Autodesk Inventor part; units mm, degrees
ref_plane "開始平面" through (0, 0, 0) normal (0, 0, 1) x (1, 0, 0)
ref_plane "終了平面" through (0, 0, 300) normal (0, 0, 1) x (1, 0, 0)
ref_plane "YZ Plane" through (0, 0, 0) normal (1, 0, 0) x (0, 1, 0)
ref_plane "開始平面" through (0, 0, 0) normal (0, 0, 1) x (1, 0, 0)
ref_plane "終了平面" through (0, 0, 300) normal (0, 0, 1) x (1, 0, 0)
sketch "スケッチ" plane through (0, 0, 0) normal (0, 0, 1) x (1, 0, 0)
  line L0 (-12.8, 0) -> (-12.8, 37.5)
  line L1 (-12.8, 37.5) -> (27.2, 37.5)
  line L2 (27.2, 37.5) -> (27.2, 35.6964)
  line L3 (23.5486, 31.7116) -> (-0.4973, 29.6078)
  line L4 (-7.8, 21.6383) -> (-7.8, 0)
  line L5 (-7.8, 0) -> (-12.8, 0) construction
  line L6 (9.7, 37.5) -> (9.7, 30.5) construction
  line L7 (27.2, 32.0311) -> (27.2, 30.5) construction
  line L8 (27.2, 30.5) -> (9.7, 30.5) construction
  line L9 (0, 15) -> (0, -27) construction
  line L10 (-5.539, 0) -> (16.0067, 0) construction
  line L11 (-12.8, 0) -> (-12.8, -37.5)
  line L12 (-12.8, -37.5) -> (27.2, -37.5)
  line L13 (27.2, -37.5) -> (27.2, -35.6964)
  line L14 (23.5486, -31.7116) -> (-0.4973, -29.6078)
  line L15 (-7.8, -21.6383) -> (-7.8, 0)
  arc A0 (-0.4973, 29.6078) -> (-7.8, 21.6383) centre (0.2, 21.6383) ccw
  arc A1 (-7.8, -21.6383) -> (-0.4973, -29.6078) centre (0.2, -21.6383) ccw
  arc A2 (23.5486, 31.7116) -> (27.2, 35.6964) centre (23.2, 35.6964) ccw
  arc A3 (27.2, -35.6964) -> (23.5486, -31.7116) centre (23.2, -35.6964) ccw
  line L16 (0, 52.5) -> (0, -52.5) construction
  line L17 (-20.955, 0) -> (36.1298, 0) construction
  point P0 (-7.8, 28.9689)
  point P1 (27.2, -32.0311)
  point P2 (-7.8, -28.9689)
  point P3 (9.7, -37.5)
  point P4 (9.7, -30.5)
  dimension "d0" = 5
  dimension "d1" = 37.5
  dimension "d2" = 40
  dimension "d3" = 7
  dimension "d4" = 17.5
  dimension "d5" = 1.5311
  dimension "d23" = 8
  dimension "d24" = 4
  dimension "d25" = 12.8
extrude "ボディ" add sketch "スケッチ" along normal up to surface (300 mm away) from surface at 0
sketch "Sketch3" plane through (0, 0, 0) normal (0, 0, 1) x (1, 0, 0)
  line L0 (0, 0) -> (10, 0)
ref_plane "Work Plane3" through (0, 0, 0) normal (0, -1, 0) x (1, 0, 0)
sketch "Sketch4" plane through (0, 0, 0) normal (0, -1, 0) x (1, 0, 0)
  line L0 (-2, 0) -> (12, 0)
  line L1 (-2, 300) -> (12, 300)
  dimension "d29" = 300
equation "\"d0\" = G_T"
equation "\"d1\" = 0.5 * G_H"
equation "\"d2\" = G_W"
equation "\"d3\" = G_T1"
equation "\"d4\" = G_C"
equation "\"d23\" = G_IR"
equation "\"d24\" = G_ER"
equation "\"d25\" = ey"
equation "\"d6\" = G_L"
equation "\"G_W\" = 40"
equation "\"G_H\" = 75"
equation "\"G_T\" = 5"
equation "\"G_T1\" = 7"
equation "\"G_NG\" = 0.08749"
equation "\"G_ER\" = 4"
equation "\"G_IR\" = 8"
equation "\"G_C\" = 17.5"
equation "\"G_L\" = d29"
equation "\"ey\" = 12.8"
equation "\"G_OFFSET_START\" = 0"
equation "\"G_OFFSET_END\" = 0"
properties part number "JIS G 3192 - 75 x 40 x 5 - 300" material "SS400"
Geometry check sheet. Reference: the model listing, model coordinates, mm. A direction names the side the tool comes from. Give positions to 0.01 mm unless a question says otherwise; leave off trailing zeros. Order: outer loops, then holes, each group sorted by start corner. A loop starts at its lowest first (then second) coordinate and runs counter-clockwise, first axis right, second up.
1. Access from +Z, -Z, +X, -X, +Y, -Y to the whole of each face (thin tool, end or side, straight path). Record for faces 5 (the face through (-9, 0, 0)), 6 (the face through (11.694, -30.674, 147.9)).
Completed:
face 5: -Z, +X, -X, +Y, -Y
face 6: +Z, -Z, +X
2. Sectioned sample at A-A (x = -3). Record the boundary of the cut face in (y, z), then the cut area to 3 significant figures.
Completed:
outline: (-37.5, 0) - (-28.97, 0) - (-28.97, 300) - (-37.5, 300) - close; (28.97, 0) - (37.5, 0) - (37.5, 300) - (28.97, 300) - close
area: 5,120 mm2
3. Draft check along Y on faces 1 (the face through (11.694, 30.674, 147.9)), 2 (the face through (-9, 0, 300)), 3 (the face through (7, -37.5, 148)), 4 (the face through (-5.754, 26.981, 147.9)). Enter one of: pulls with the +Y half, pulls with the -Y half, needs draft (parallel to the pull), parting line crosses it, or undercut.
Completed:
face 1: undercut
face 2: needs draft
face 3: pulls with the -Y half
face 4: undercut
4. Depth check by flat-ended pin: pin 1 (4 mm diameter, centred on y = -23.5, z = 160, fed in from +X). Enter the tip coordinate at first touch or a pass-through.
Completed:
pin 1: stops at x = -6.81
5. Sectioned sample at C-C (y = 14.5). Record the boundary of the cut face in (x, z), then the cut area to 3 significant figures.
Completed:
outline: (-12.8, 0) - (-7.8, 0) - (-7.8, 300) - (-12.8, 300) - close
area: 1,500 mm2
6. Sectioned sample at B-B (z = 198). Record the boundary of the cut face in (x, y).
Completed:
outline: (-12.8, -37.5) - (27.2, -37.5) - (27.2, -35.7) arc R4 ccw to (23.55, -31.71) - (-0.5, -29.61) arc R8 cw to (-7.8, -21.64) - (-7.8, 21.64) arc R8 cw to (-0.5, 29.61) - (23.55, 31.71) arc R4 ccw to (27.2, 35.7) - (27.2, 37.5) - (-12.8, 37.5) - close
7. Scan lines: line 1 (Y direction, x = 23.5, z = 113.5); line 2 (X direction, y = -2, z = 195.5); line 3 (Y direction, x = 12.5, z = 280.5). Record each from-to range of solid material in increasing order.
Completed:
line 1: y = -37.5 to -31.71, 31.71 to 37.5
line 2: x = -12.8 to -7.8
line 3: y = -37.5 to -30.74, 30.74 to 37.5
8. Sectioned sample at D-D (x = 8). Record the boundary of the cut face in (y, z).
Completed:
outline: (-37.5, 0) - (-30.35, 0) - (-30.35, 300) - (-37.5, 300) - close; (30.35, 0) - (37.5, 0) - (37.5, 300) - (30.35, 300) - close
